Model file for the job. Use its own axes, mm. Face numbers are marked on the shaded views. A direction names the side the tool comes from. Give positions to 0.01 mm unless a question says otherwise; leave off trailing zeros. Order: outer loops, then holes, each group sorted by start corner. A loop starts at its lowest first (then second) coordinate and runs counter-clockwise, first axis right, second up. Notation, with made-up numbers: M 54.5,73 L 105.5,73 A17 cw 105.5,90 Z; hole C -40,26 d2. An arc over 180 degrees is marked long. Return JSON: item names as keys, results as strings. Group by question number.
1. Pin check, flat tips, straight feed: pin 1 (1 mm diameter, centred on x = -0.5, z = 7.5, fed in from -Y); pin 2 (1.8 mm diameter, centred on x = -1, z = -1, fed in from +Y); pin 3 (3 mm diameter, centred on y = 2, z = -3, fed in from -X); pin 4 (4 mm diameter, centred on x = 0, z = -7.5, fed in from +Y). Stop position of each tip, or through.
2. Two-plate mould, pull along X, no slides. Class the marked faces 3, 4 and 5: released by +X, released by -X, zero draft, split by the parting line, or undercut.
3. 3-axis set-ups, long thin cutter, end or side, ignore diameter. For the marked faces 1 and 2: which of +Z, -Z, +X, -X, +Y, -Y reach the whole face in a straight line?
4. Slice it at C-C on y = 2.25. List the corners of the cut face in (x, z).
5. Slice it at D-D on x = 7.5. List the corners of the cut face in (y, z), then the cut area to 3 significant figures.
6. Wall check: probe 1 along X at (y, z) = (0.5, -1); probe 2 along Y at (x, z) = (7, 2.25); probe 3 along Z at (x, y) = (0, 4.65). Give the ranges that are in metal, low to high. Write a range as [from, to].
7. Slice it at B-B on z = 7.5. List the corners of the cut face in (x, y).
8. Slice it at A-A on x = 0. List the corners of the cut face in (y, z).
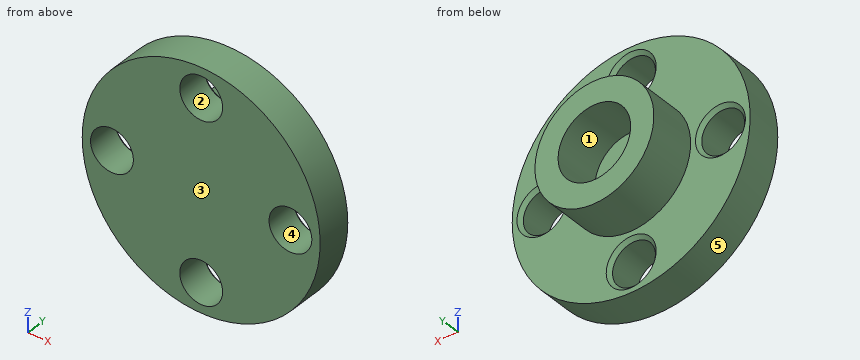
Autodesk Inventor part; units mm, degrees
ref_plane "YZ Plane" through (0, 0, 0) normal (1, 0, 0) x (0, 1, 0)
ref_plane "XZ Plane" through (0, 0, 0) normal (0, 1, 0) x (-1, 0, 0)
ref_plane "XY Plane" through (0, 0, 0) normal (0, 0, 1) x (1, 0, 0)
sketch "Эскиз1" plane through (0, 0, 0) normal (0, 1, 0) x (-1, 0, 0)
  circle A0 centre (0, 0) radius 10
  dimension "d0" = 20
extrude "Выдавливание1" add sketch "Эскиз1" along normal blind 3
sketch "Эскиз2" plane through (0, 3, 0) normal (0, 1, 0) x (1, 0, 0)
  circle A0 centre (0, 0) radius 10
  circle A1 centre (0, 0) radius 5
  dimension "d3" = 10
extrude "Выдавливание2" add sketch "Эскиз2" along normal blind 4 contours A1
sketch "Эскиз3" plane through (0, 7, 0) normal (0, 1, 0) x (1, 0, 0)
  circle A0 centre (0, 0) radius 5
hole "Отверстие1" at (0, 7, 0) direction (0, -1, 0) diameter 6.1 depth 4
sketch "Эскиз4" plane through (0, 3, 0) normal (0, 1, 0) x (1, 0, 0)
  circle A0 centre (0, 0) radius 5
  circle A1 centre (0, 0) radius 10
  circle A2 centre (0, 0) radius 7.5 construction
  point P0 (0, -7.5)
  dimension "d22" = 15
  dimension "d13" = 5
hole "Отверстие2" at (0, 3, 7.5) direction (0, -1, 0) diameter 3.6 depth 4 countersink diameter 4.2 countersink angle 90
pattern_circular "Круговой массив1" count 4 over 360 about axis through (0, 5, 0) along (0, 1, 0) of "Отверстие2"
properties part number "втулка"
Result:
{
 "1": {"pin 1": "passes through", "pin 2": "stops at y = 3", "pin 3": "stops at x = -9.89", "pin 4": "stops at y = 2.9"},
 "2": {"face 3": "zero draft", "face 4": "undercut", "face 5": "split by the parting line"},
 "3": {"face 1": "+Y", "face 2": "+Y, -Y"},
 "4": {"outline": "C 0,0 d20; hole C -7.5,0 d3.6; hole C 0,-7.5 d3.6; hole C 0,7.5 d3.6; hole C 7.5,0 d3.6"},
 "5": {"outline": "M 0,-6.61 L 3,-6.61 L 3,-2.1 L 2.7,-1.8 L 0,-1.8 Z; M 0,1.8 L 2.7,1.8 L 3,2.1 L 3,6.61 L 0,6.61 Z", "area": "28.8 mm2"},
 "6": {"probe 1": "x = [-9.95, -9], [-6, 6], [9, 9.95]", "probe 2": "y = [0, 3]", "probe 3": "z = [-5, -3.05], [3.05, 5]"},
 "7": {"outline": "M -6.61,0 L -1.8,0 L -1.8,2.7 L -2.1,3 L -6.61,3 Z; M 1.8,0 L 6.61,0 L 6.61,3 L 2.1,3 L 1.8,2.7 Z"},
 "8": {"outline": "M 0,-10 L 3,-10 L 3,-9.6 L 2.7,-9.3 L 0,-9.3 Z; M 0,-5.7 L 2.7,-5.7 L 3,-5.4 L 3,-5 L 7,-5 L 7,-3.05 L 3,-3.05 L 3,3.05 L 7,3.05 L 7,5 L 3,5 L 3,5.4 L 2.7,5.7 L 0,5.7 Z; M 0,9.3 L 2.7,9.3 L 3,9.6 L 3,10 L 0,10 Z"}
}
